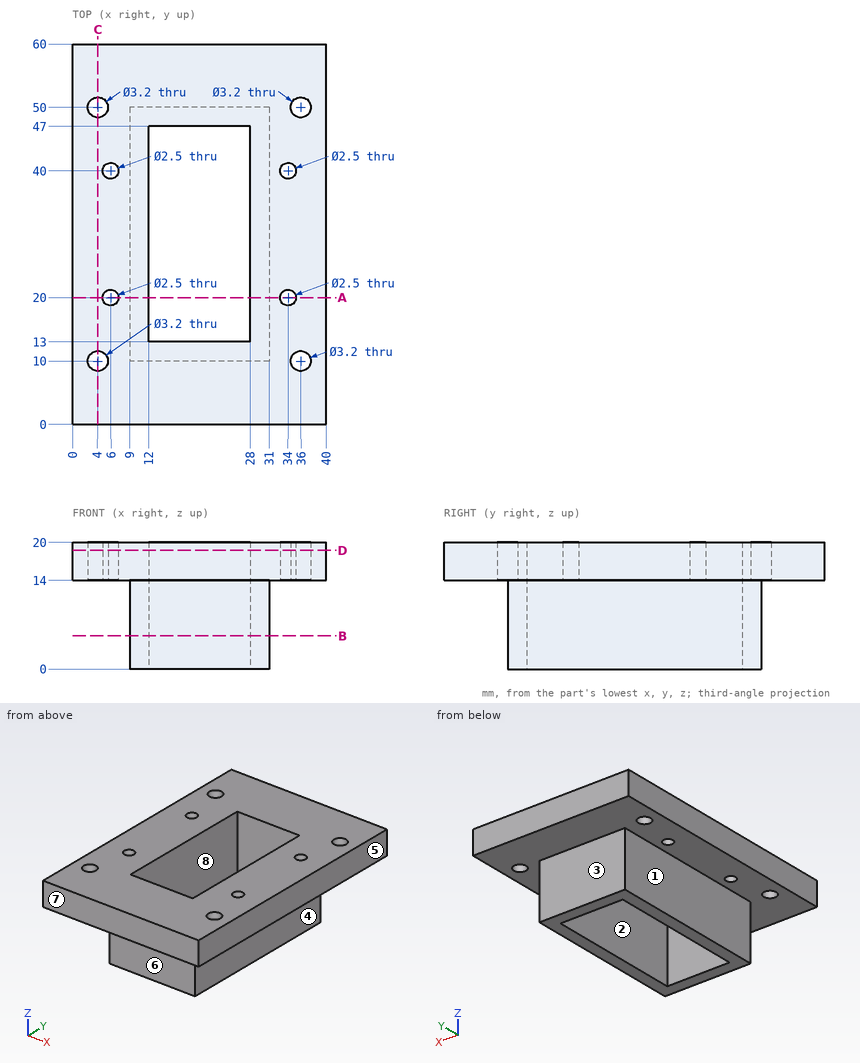
Check sheet for the drawn part. Datum: minimum x, y, z corner. Units: mm. A direction names the side the tool comes from. Give positions to 0.01 mm unless a question says otherwise; leave off trailing zeros. Loops run counter-clockwise (first coordinate to the right, second up) from the corner with the lowest first, then second, coordinate; pieces in that order, holes last. Notation, with made-up numbers: M 47.25,78.5 L 84.25,78.5 A7 cw 84.25,87.5 Z; hole C -21.75,-26 d10. An arc over 180 degrees is marked long. Answer as CSV lines item,"result".
Item 1: Depth check by flat-ended pin: pin 1 Ø6 at (x, y) = (11.5, 26) entering from -Z; pin 2 Ø3 at (x, y) = (34, 40) entering from -Z; pin 3 Ø10 at (y, z) = (35.5, 6.5) entering from +X; pin 4 Ø7 at (x, z) = (19.5, 5) entering from -Y. Enter the tip coordinate at first touch or a pass-through.
Reply:
pin 1,"z = 0"
pin 2,"z = 14"
pin 3,"x = 31"
pin 4,"y = 10"
Item 2: Sectioned sample at A-A, the plane y = 20. Enter the section's corners in (x, z).
Reply:
outline,"M 0,14 L 4.75,14 L 4.75,20 L 0,20 Z; M 7.25,14 L 9,14 L 9,0 L 12,0 L 12,20 L 7.25,20 Z; M 28,0 L 31,0 L 31,14 L 32.75,14 L 32.75,20 L 28,20 Z; M 35.25,14 L 40,14 L 40,20 L 35.25,20 Z"
Item 3: Set-up check for the marked faces 4, 5, 6, 7 and 8: record each of +Z, -Z, +X, -X, +Y, -Y from which the full face is reachable in a straight line by a thin tool's end or side.
Reply:
face 4,"-Z, +X, +Y, -Y"
face 5,"+Z, -Z, +X, +Y, -Y"
face 6,"-Z, +X, -X, -Y"
face 7,"+Z, -Z, +X, -X, -Y"
face 8,"+Z, -Z"
Item 4: Sectioned sample at C-C, the plane x = 4. Enter the section's corners in (y, z).
Reply:
outline,"M 0,14 L 8.4,14 L 8.4,20 L 0,20 Z; M 11.6,14 L 48.4,14 L 48.4,20 L 11.6,20 Z; M 51.6,14 L 60,14 L 60,20 L 51.6,20 Z"
Item 5: Scan lines: L1, parallel to Y at x = 36, z = 16.7; L2, parallel to X at y = 46, z = 17.5; L3, parallel to Y at x = 21, z = 1.25. Record each from-to range of solid material in increasing order.
Reply:
L1,"0 to 8.4, 11.6 to 48.4, 51.6 to 60"
L2,"0 to 12, 28 to 40"
L3,"10 to 13, 47 to 50"
Item 6: Sectioned sample at D-D, the plane z = 18.75. State how many separate pieces and enclosed holes the cut face has, then the cut area to 3 significant figures.
Reply:
separate pieces,"1"
enclosed holes,"9"
area,"1,800 mm^2"
Item 7: Sectioned sample at B-B, the plane z = 5.25. Enter the section's corners in (x, y).
Reply:
outline,"M 9,10 L 31,10 L 31,50 L 9,50 Z; hole M 12,13 L 28,13 L 28,47 L 12,47 Z"
Item 8: Draft check along Y on the marked faces 1, 2 and 3. Enter one of: pulls with the +Y half, pulls with the -Y half, needs draft (parallel to the pull), parting line crosses it, or undercut.
Reply:
face 1,"needs draft"
face 2,"undercut"
face 3,"pulls with the +Y half"
